Source: CAD feature listing. Evaluate the final solid. Frame: model axes, mm. Face numbers are marked on the shaded views. A direction names the side the tool comes from. Coordinates: 2 decimals unless noted, no trailing zeros. Loops run counter-clockwise (first coordinate to the right, second up) from the corner with the lowest first, then second, coordinate; pieces in that order, holes last.
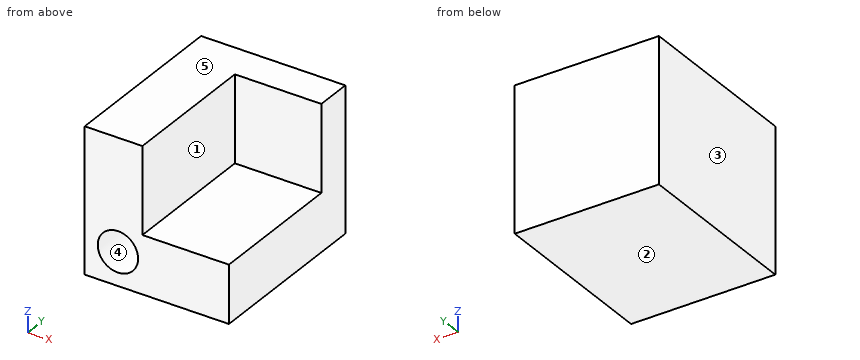
from build123d import *

# Parameters (mm, degrees)
SKETCH1_R           = 1.4
BOSS_EXTRUDE1_DEPTH = 9.65
SKETCH2_W           = 10
SKETCH2_H           = 10
BOSS_EXTRUDE2_DEPTH = 2.5


with BuildPart() as part:
    # Sketch1 → Boss-Extrude1 (new body)
    with BuildSketch(Plane(origin=(0, 0, 0), x_dir=(1, 0, 0), z_dir=(0, 1, 0))):
        Polygon((0, 0), (10, 0), (10, -4), (4, -4), (4, -10), (0, -10), align=None)
        with Locations(Location((2.302943725, -2.302943725, 0), (0, 0, 270))):
            Circle(SKETCH1_R, mode=Mode.SUBTRACT)
    extrude(amount=BOSS_EXTRUDE1_DEPTH)

    # Sketch2 → Boss-Extrude2 (add)
    with BuildSketch(Plane(origin=(0, 9.65, 0), x_dir=(1, 0, 0), z_dir=(0, 1, 0))):
        with Locations((5, -5)):
            Rectangle(SKETCH2_W, SKETCH2_H)
    extrude(amount=BOSS_EXTRUDE2_DEPTH)


solid = part.part
Q1. Section C-C, the plane y = 6. Return the cut outline in (x, z).
Q2. Section A-A, the plane x = 5.5. Return the cut outline in (y, z), plus the area to 3 significant figures.
Q3. Access query for the marked faces 1 and 2. Directions: +Z, -Z, +X, -X, +Y, -Y. A direction counts if a zero-diameter tool reaches every point of the face in a straight line with its end or side. Return the directions, or none.
Q4. Draft query along X for the marked faces 3, 4 and 5. Return one class per face: +X half, -X half, draft (parallel to the pull), parting line (faces both ways), or undercut.
Q5. Section B-B, the plane z = 2.5. Return the cut outline in (x, y).
Q6. Contact query for flat-ended pins moving along their axis: pin 1 Ø3 at (x, z) = (7.5, 7.5) entering from -Y; pin 2 Ø4 at (x, y) = (2.5, 9) entering from -Z; pin 3 Ø3 at (x, y) = (6, 5) entering from +Z. Output: stop coordinate, or through.
Q7. Section D-D, the plane x = 2.75. Return the cut outline in (y, z), plus the area to 3 significant figures.
Q8. Line query: line 1 along Y through (x, z) = (4.75, 7.5); line 2 along X through (y, z) = (5.75, 4.75). Output: solid intervals per line, ascending.
Derived:
1. outline: (0, 0) - (10, 0) - (10, 4) - (4, 4) - (4, 10) - (0, 10) - close; hole circle Ø2.8 at (2.3, 2.3)
2. outline: (0, 0) - (12.15, 0) - (12.15, 10) - (9.65, 10) - (9.65, 4) - (0, 4) - close
2. area: 63.6 mm2
3. face 1: +Z, +X, -Y
3. face 2: -Z, +X, -X, +Y, -Y
4. face 3: -X half
4. face 4: undercut
4. face 5: draft
5. outline: (0, 0) - (0.92, 0) - (0.92, 9.65) - (3.69, 9.65) - (3.69, 0) - (10, 0) - (10, 12.15) - (0, 12.15) - close
6. pin 1: stops at y = 9.65
6. pin 2: stops at z = 0
6. pin 3: stops at z = 4
7. outline: (0, 0) - (12.15, 0) - (12.15, 10) - (0, 10) - (0, 3.63) - (9.65, 3.63) - (9.65, 0.98) - (0, 0.98) - close
7. area: 95.9 mm2
8. line 1: y = 9.65 to 12.15
8. line 2: x = 0 to 4
